```python
from build123d import *

# Parameters (mm, degrees)
ESQUISSE1_W             = 22.098
ESQUISSE1_H             = 33.782
BOSS_EXTRU_1_DEPTH      = 1.048
ESQUISSE2_W             = 19.05
ESQUISSE2_H             = 23.442994478
BOSS_EXTRU_2_DEPTH      = 2
ENL_V_MAT_EXTRU_1_DEPTH = 2
CONG_1_R                = 0.25


with BuildPart() as part:
    # Esquisse1 → Boss.-Extru.1 (new body)
    with BuildSketch(Plane(origin=(0, 0, 0), x_dir=(1, 0, 0), z_dir=(0, 1, 0))):
        with Locations((11.049, 16.891)):
            Rectangle(ESQUISSE1_W, ESQUISSE1_H)
    extrude(amount=BOSS_EXTRU_1_DEPTH)

    # Esquisse2 → Boss.-Extru.2 (add)
    with BuildSketch(Plane(origin=(0, 1.048, 0), x_dir=(1, 0, 0), z_dir=(0, 1, 0))):
        with Locations((11.049, 13.245497239)):
            Rectangle(ESQUISSE2_W, ESQUISSE2_H)
    extrude(amount=BOSS_EXTRU_2_DEPTH)

    # Esquisse3 → Enlèv. mat.-Extru.1 (cut)
    with BuildSketch(Plane(origin=(0, 1.048, 0), x_dir=(1, 0, 0), z_dir=(0, 1, 0))):
        with BuildLine():
            Line((0, 26.4604), (0, 25.6604))
            ThreePointArc((0, 25.6604), (0.4, 26.0604), (0, 26.4604))
        make_face()
        with BuildLine():
            Line((22.098, 26.4604), (22.098, 25.6604))
            ThreePointArc((22.098, 25.6604), (21.698, 26.0604), (22.098, 26.4604))
        make_face()
        with BuildLine():
            Line((22.098, 24.4004), (22.098, 23.6004))
            ThreePointArc((22.098, 23.6004), (21.698, 24.0004), (22.098, 24.4004))
        make_face()
        with BuildLine():
            Line((0, 24.4004), (0, 23.6004))
            ThreePointArc((0, 23.6004), (0.4, 24.0004), (0, 24.4004))
        make_face()
        with BuildLine():
            Line((22.098, 22.3404), (22.098, 21.5404))
            ThreePointArc((22.098, 21.5404), (21.698, 21.9404), (22.098, 22.3404))
        make_face()
        with BuildLine():
            Line((0, 22.3404), (0, 21.5404))
            ThreePointArc((0, 21.5404), (0.4, 21.9404), (0, 22.3404))
        make_face()
        with BuildLine():
            Line((22.098, 20.2804), (22.098, 19.4804))
            ThreePointArc((22.098, 19.4804), (21.698, 19.8804), (22.098, 20.2804))
        make_face()
        with BuildLine():
            Line((0, 20.2804), (0, 19.4804))
            ThreePointArc((0, 19.4804), (0.4, 19.8804), (0, 20.2804))
        make_face()
        with BuildLine():
            Line((22.098, 18.2204), (22.098, 17.4204))
            ThreePointArc((22.098, 17.4204), (21.698, 17.8204), (22.098, 18.2204))
        make_face()
        with BuildLine():
            Line((0, 18.2204), (0, 17.4204))
            ThreePointArc((0, 17.4204), (0.4, 17.8204), (0, 18.2204))
        make_face()
        with BuildLine():
            Line((22.098, 16.1604), (22.098, 15.3604))
            ThreePointArc((22.098, 15.3604), (21.698, 15.7604), (22.098, 16.1604))
        make_face()
        with BuildLine():
            Line((0, 16.1604), (0, 15.3604))
            ThreePointArc((0, 15.3604), (0.4, 15.7604), (0, 16.1604))
        make_face()
        with BuildLine():
            Line((22.098, 14.1004), (22.098, 13.3004))
            ThreePointArc((22.098, 13.3004), (21.698, 13.7004), (22.098, 14.1004))
        make_face()
        with BuildLine():
            Line((0, 14.1004), (0, 13.3004))
            ThreePointArc((0, 13.3004), (0.4, 13.7004), (0, 14.1004))
        make_face()
        with BuildLine():
            Line((22.098, 12.0404), (22.098, 11.2404))
            ThreePointArc((22.098, 11.2404), (21.698, 11.6404), (22.098, 12.0404))
        make_face()
        with BuildLine():
            Line((0, 12.0404), (0, 11.2404))
            ThreePointArc((0, 11.2404), (0.4, 11.6404), (0, 12.0404))
        make_face()
        with BuildLine():
            Line((22.098, 9.9804), (22.098, 9.1804))
            ThreePointArc((22.098, 9.1804), (21.698, 9.5804), (22.098, 9.9804))
        make_face()
        with BuildLine():
            Line((0, 9.9804), (0, 9.1804))
            ThreePointArc((0, 9.1804), (0.4, 9.5804), (0, 9.9804))
        make_face()
        with BuildLine():
            Line((22.098, 7.9204), (22.098, 7.1204))
            ThreePointArc((22.098, 7.1204), (21.698, 7.5204), (22.098, 7.9204))
        make_face()
        with BuildLine():
            Line((0, 7.9204), (0, 7.1204))
            ThreePointArc((0, 7.1204), (0.4, 7.5204), (0, 7.9204))
        make_face()
        with BuildLine():
            Line((22.098, 5.8604), (22.098, 5.0604))
            ThreePointArc((22.098, 5.0604), (21.698, 5.4604), (22.098, 5.8604))
        make_face()
        with BuildLine():
            Line((0, 5.8604), (0, 5.0604))
            ThreePointArc((0, 5.0604), (0.4, 5.4604), (0, 5.8604))
        make_face()
        with BuildLine():
            Line((22.098, 3.8004), (22.098, 3.0004))
            ThreePointArc((22.098, 3.0004), (21.698, 3.4004), (22.098, 3.8004))
        make_face()
        with BuildLine():
            Line((0, 3.8004), (0, 3.0004))
            ThreePointArc((0, 3.0004), (0.4, 3.4004), (0, 3.8004))
        make_face()
        with BuildLine():
            Line((22.098, 1.7404), (22.098, 0.9404))
            ThreePointArc((22.098, 0.9404), (21.698, 1.3404), (22.098, 1.7404))
        make_face()
        with BuildLine():
            Line((0, 1.7404), (0, 0.9404))
            ThreePointArc((0, 0.9404), (0.4, 1.3404), (0, 1.7404))
        make_face()
        with BuildLine():
            Line((22.098, 28.5204), (22.098, 27.7204))
            ThreePointArc((22.098, 27.7204), (21.698, 28.1204), (22.098, 28.5204))
        make_face()
        with BuildLine():
            Line((22.098, 30.5804), (22.098, 29.7804))
            ThreePointArc((22.098, 29.7804), (21.698, 30.1804), (22.098, 30.5804))
        make_face()
        with BuildLine():
            Line((22.098, 32.6404), (22.098, 31.8404))
            ThreePointArc((22.098, 31.8404), (21.698, 32.2404), (22.098, 32.6404))
        make_face()
        with BuildLine():
            Line((10.419, 0), (9.619, 0))
            ThreePointArc((9.619, 0), (10.019, 0.4), (10.419, 0))
        make_face()
        with BuildLine():
            Line((12.479, 0), (11.679, 0))
            ThreePointArc((11.679, 0), (12.079, 0.4), (12.479, 0))
        make_face()
        with BuildLine():
            Line((14.539, 0), (13.739, 0))
            ThreePointArc((13.739, 0), (14.139, 0.4), (14.539, 0))
        make_face()
        with BuildLine():
            Line((16.599, 0), (15.799, 0))
            ThreePointArc((15.799, 0), (16.199, 0.4), (16.599, 0))
        make_face()
        with BuildLine():
            Line((18.659, 0), (17.859, 0))
            ThreePointArc((17.859, 0), (18.259, 0.4), (18.659, 0))
        make_face()
        with BuildLine():
            Line((8.359, 0), (7.559, 0))
            ThreePointArc((7.559, 0), (7.959, 0.4), (8.359, 0))
        make_face()
        with BuildLine():
            Line((6.299, 0), (5.499, 0))
            ThreePointArc((5.499, 0), (5.899, 0.4), (6.299, 0))
        make_face()
        with BuildLine():
            Line((4.239, 0), (3.439, 0))
            ThreePointArc((3.439, 0), (3.839, 0.4), (4.239, 0))
        make_face()
    extrude(amount=-ENL_V_MAT_EXTRU_1_DEPTH, mode=Mode.SUBTRACT)

    # Congé1
    cong_1_edges = [part.edges().sort_by_distance(p)[0] for p in [
        (1.524, 2.048, -24.966994478),
        (1.524, 2.048, -1.524),
        (20.574, 2.048, -1.524),
        (20.574, 2.048, -24.966994478),
        (1.524, 3.048, -13.245497239),
        (11.049, 3.048, -1.524),
        (20.574, 3.048, -13.245497239),
        (11.049, 3.048, -24.966994478),
    ]]
    fillet(cong_1_edges, radius=CONG_1_R)


solid = part.part
```
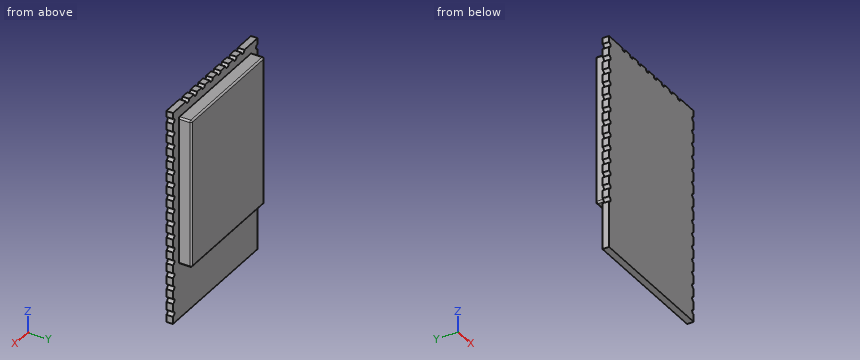
Geometry check sheet. Reference: the model listing, model coordinates, mm. Round coordinates to 2 decimals unless told otherwise and drop trailing zeros. Loops run counter-clockwise (first coordinate to the right, second up) from the corner with the lowest first, then second, coordinate; pieces in that order, holes last. Notation, with made-up numbers: M 19.5,49 L 26.5,49 A20 cw 26.5,60 Z; hole C -7,-11.75 d9. An arc over 180 degrees is marked long. Return JSON: item names as keys, results as strings. Group by question number.
(1) Section check C-C, the plane z = -19. Enter the section's corners in (x, y), and give its area (3 significant figures).
(2) Scan lines: line 1 along X through (y, z) = (2.2, -10.5); line 2 along Z through (x, y) = (10.25, 1.25); line 3 along Y through (x, z) = (9.75, -30). Record each from-to range of solid material in increasing order. Write a range as [from, to].
(3) Section check A-A, the plane y = 1.95. Enter the section's corners in (x, z).
(4) Go/stop test with flat-tipped pins: pin 1 (1.4 mm diameter, centred on y = 2, z = -19, fed in from +X); pin 2 (0.5 mm diameter, centred on x = 10.5, y = 1.5, fed in from -Z). Record where each tip stops, or that it passes through.
(5) Section check B-B, the plane x = 19.75. Enter the section's corners in (y, z).
(6) Section check D-D, the plane z = -26. Enter the section's corners in (x, y).
Data:
{
 "1": {"outline": "M 0,0 L 22.1,0 L 22.1,1.05 L 20.57,1.05 L 20.57,2.8 A0.25 ccw 20.32,3.05 L 1.77,3.05 A0.25 ccw 1.52,2.8 L 1.52,1.05 L 0,1.05 Z", "area": "61.2 mm²"},
 "2": {"line 1": "[1.52, 20.57]", "line 2": "[-24.97, -1.52]", "line 3": "[0, 1.05]"},
 "3": {"outline": "M 1.52,-24.72 A0.25 ccw 1.77,-24.97 L 20.32,-24.97 A0.25 ccw 20.57,-24.72 L 20.57,-1.77 A0.25 ccw 20.32,-1.52 L 1.77,-1.52 A0.25 ccw 1.52,-1.77 Z"},
 "4": {"pin 1": "x = 20.57", "pin 2": "z = -24.97"},
 "5": {"outline": "M 0,-33.78 L 1.05,-33.78 L 1.05,-24.97 L 2.8,-24.97 A0.25 ccw 3.05,-24.72 L 3.05,-1.77 A0.25 ccw 2.8,-1.52 L 1.05,-1.52 L 1.05,0 L 0,0 Z"},
 "6": {"outline": "M 0.4,0 L 21.7,0 L 21.7,1.05 L 0.4,1.05 Z"}
}
